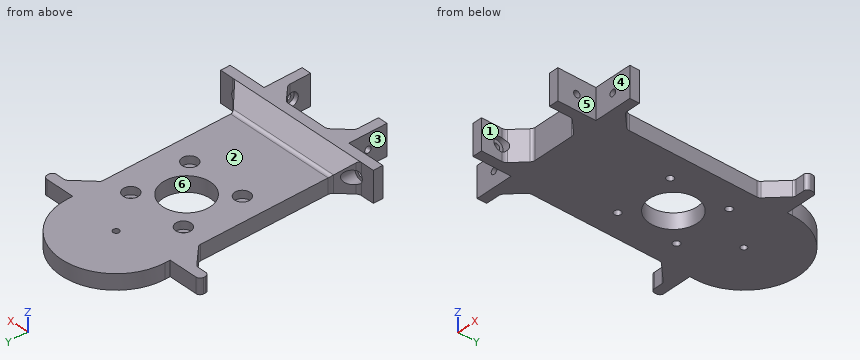
from build123d import *

# Parameters (mm, degrees)
RESSALTO_EXTRUS_O1_DEPTH                     = 8
RESSALTO_EXTRUS_O2_DEPTH                     = 8
CHANFRO1_SIZE                                = 8
ESBO_O3_R                                    = 1.6
ESBO_O3_R_2                                  = 12.5
CORTE_EXTRUS_O1_DEPTH                        = 138.275962936
FILETE1_R                                    = 3
REBAIXO_PARA_PARAFUSO_COM_CABE_A_PAN_2_COUNT = 2
REBAIXO_PARA_PARAFUSO_COM_CABE_A_PAN_2_PITCH = 70
CORTE_EXTRUS_O3_START                        = 10
ESBO_O13_R                                   = 3.5
CORTE_EXTRUS_O3_DEPTH                        = 10
ESBO_O18_R                                   = 3.5
CORTE_EXTRUS_O4_DEPTH                        = 2
ESBO_O19_R                                   = 1.8
CORTE_EXTRUS_O5_DEPTH                        = 137.574851278
ESBO_O20_R                                   = 4
CORTE_EXTRUS_O6_DEPTH                        = 4
ESBO_O21_W                                   = 17.35
ESBO_O21_H                                   = 5
RESSALTO_EXTRUS_O3_DEPTH                     = 8
FILETE2_R                                    = 2
CHANFRO2_SIZE                                = 10
FILETE3_R                                    = 2


with BuildPart() as part:
    # Esboço1 → Ressalto-extrusão1 (new body)
    with BuildSketch(Plane.XY):
        with BuildLine():
            Line((28.7, 5), (28.7, 100))
            ThreePointArc((28.7, 100), (0, 128.7), (-28.7, 100))
            Line((-28.7, 100), (-28.7, 5))
            Line((-28.7, 5), (-45, 5))
            Line((-45, 5), (-45, 0))
            Line((-45, 0), (-25, 0))
            Line((-25, 0), (-25, -20))
            Line((-25, -20), (-20, -20))
            Line((-20, -20), (-20, 0))
            Line((-20, 0), (20, 0))
            Line((20, 0), (20, -20))
            Line((20, -20), (25, -20))
            Line((25, -20), (25, 0))
            Line((25, 0), (45, 0))
            Line((45, 0), (45, 5))
            Line((45, 5), (28.7, 5))
        make_face()
    extrude(amount=RESSALTO_EXTRUS_O1_DEPTH)

    # Esboço2 → Ressalto-extrusão2 (add)
    with BuildSketch(Plane.XY.offset(8)):
        Polygon((-20, -20), (-25, -20), (-25, 0), (-45, 0), (-45, 5), (45, 5), (45, 0), (25, 0), (25, -20), (20, -20), (20, 0), (-20, 0), align=None)
    extrude(amount=RESSALTO_EXTRUS_O2_DEPTH)

    # Chanfro1
    chanfro1_edges = [part.edges().sort_by_distance(p)[0] for p in [
        (28.7, 5, 4),
        (20, 0, 8),
        (-20, 0, 8),
        (-28.7, 5, 4),
        (0, 5, 8),
    ]]
    chamfer(chanfro1_edges, length=CHANFRO1_SIZE - 0.0001)  # a hair under: the kernel refuses the full size

    # Esboço3 → Corte-extrusão1 (cut, through all)
    with BuildSketch(Plane(origin=(0, 0, 0), x_dir=(-1, 0, 0), z_dir=(0, 0, -1))):
        with Locations((0, 100)):
            Circle(ESBO_O3_R)
        with Locations((0, 63)):
            Circle(ESBO_O3_R_2)
    extrude(amount=-CORTE_EXTRUS_O1_DEPTH, mode=Mode.SUBTRACT)

    # Filete1
    filete1_edges = [part.edges().sort_by_distance(p)[0] for p in [
        (28.7, 12.9999, 4),
        (-36.6999, 5, 7.99995),
        (36.6999, 5, 7.99995),
        (-28.7, 12.9999, 4),
        (0, 12.9999, 8),
        (20, -7.9999, 8),
        (-12.0001, 0, 8),
        (12.0001, 0, 8),
        (-20, -7.9999, 8),
    ]]
    fillet(filete1_edges, radius=FILETE1_R)

    # Esboço12 → Rebaixo para parafuso com cabe_a panela (revolve, cut)
    with BuildSketch(Plane(origin=(35, 5, 8), x_dir=(0, 0, 1), z_dir=(1, 0, 0))):
        Polygon((0, 0), (0, 7.021463052), (1.7, 6), (1.7, 2.4), (3.5, 2.4), (3.5, 0), align=None)
    rebaixo_para_parafuso_com_cabe_a_panela = revolve(axis=Axis((35, 11.35, 8), (0, -1, 0)), mode=Mode.SUBTRACT)

    # Rebaixo para parafuso com cabe_a pan 2: Rebaixo para parafuso com cabe_a panela ×2
    with Locations(*[(-i * REBAIXO_PARA_PARAFUSO_COM_CABE_A_PAN_2_PITCH, 0, 0) for i in range(1, REBAIXO_PARA_PARAFUSO_COM_CABE_A_PAN_2_COUNT)]):
        add(rebaixo_para_parafuso_com_cabe_a_panela, mode=Mode.SUBTRACT)

    # Esboço13 → Corte-extrusão3 (cut)
    with BuildSketch(Plane(origin=(0, 5, 0), x_dir=(1, 0, 0), z_dir=(0, 1, 0)).offset(CORTE_EXTRUS_O3_START)):
        with Locations(Location((-35, -8, 0), (0, 0, 270))):
            Circle(ESBO_O13_R)
        with Locations(Location((35, -8, 0), (0, 0, 270))):
            Circle(ESBO_O13_R)
    extrude(amount=-CORTE_EXTRUS_O3_DEPTH, mode=Mode.SUBTRACT)

    # Esboço15 → Rebaixo para parafuso com cabe_a pan 3 (revolve, cut)
    with BuildSketch(Plane(origin=(20, -10, 8), x_dir=(0, 0, 1), z_dir=(0, 1, 0))):
        Polygon((0, 0), (0, 7.021463052), (1.7, 6), (1.7, 2.4), (3.5, 2.4), (3.5, 0), align=None)
    revolve(axis=Axis((13.65, -10, 8), (1, 0, 0)), mode=Mode.SUBTRACT)

    # Esboço17 → Rebaixo para parafuso com cabe_a pan 4 (revolve, cut)
    with BuildSketch(Plane(origin=(-20, -10, 8), x_dir=(0, 0, -1), z_dir=(0, 1, 0))):
        Polygon((0, 0), (0, 7.021463052), (1.7, 6), (1.7, 2.4), (3.5, 2.4), (3.5, 0), align=None)
    revolve(axis=Axis((-13.65, -10, 8), (-1, 0, 0)), mode=Mode.SUBTRACT)

    # Esboço18 → Corte-extrusão4 (cut)
    with BuildSketch(Plane.ZY.offset(-20)):
        with Locations((8, -10)):
            Circle(ESBO_O18_R)
    corte_extrus_o4 = extrude(amount=CORTE_EXTRUS_O4_DEPTH, mode=Mode.SUBTRACT)

    # Espelhar1: Corte-extrusão4 across plane
    add(corte_extrus_o4.mirror(Plane(origin=(0, 0, 0), x_dir=(0, 0, 1), z_dir=(1, 0, 0))), mode=Mode.SUBTRACT)

    # Esboço19 → Corte-extrusão5 (cut, through all)
    with BuildSketch(Plane.XY.offset(8)):
        with Locations((15.5, 78.5)):
            Circle(ESBO_O19_R)
        with Locations((15.5, 47.5)):
            Circle(ESBO_O19_R)
        with Locations((-15.5, 47.5)):
            Circle(ESBO_O19_R)
        with Locations((-15.5, 78.5)):
            Circle(ESBO_O19_R)
    extrude(amount=-CORTE_EXTRUS_O5_DEPTH, mode=Mode.SUBTRACT)

    # Esboço20 → Corte-extrusão6 (cut)
    with BuildSketch(Plane.XY.offset(8)):
        with Locations((15.5, 78.5)):
            Circle(ESBO_O20_R)
        with Locations((15.5, 47.5)):
            Circle(ESBO_O20_R)
        with Locations((-15.5, 47.5)):
            Circle(ESBO_O20_R)
        with Locations((-15.5, 78.5)):
            Circle(ESBO_O20_R)
    extrude(amount=-CORTE_EXTRUS_O6_DEPTH, mode=Mode.SUBTRACT)

    # Esboço21 → Ressalto-extrusão3 (add)
    with BuildSketch(Plane(origin=(0, 0, 0), x_dir=(-1, 0, 0), z_dir=(0, 0, -1))):
        with Locations((-37.375, 94.7)):
            Rectangle(ESBO_O21_W, ESBO_O21_H)
        with Locations((37.375, 94.7)):
            Rectangle(ESBO_O21_W, ESBO_O21_H)
    extrude(amount=-RESSALTO_EXTRUS_O3_DEPTH)

    # Filete2
    filete2_edges = [part.edges().sort_by_distance(p)[0] for p in [
        (46.05, 97.2, 4),
        (46.05, 92.2, 4),
        (-46.05, 92.2, 4),
        (-46.05, 97.2, 4),
    ]]
    fillet(filete2_edges, radius=FILETE2_R)

    # Chanfro2
    chanfro2_edges = [part.edges().sort_by_distance(p)[0] for p in [
        (28.7, 92.2, 4),
        (-28.7, 92.2, 4),
    ]]
    chamfer(chanfro2_edges, length=CHANFRO2_SIZE)

    # Filete3
    filete3_edges = [part.edges().sort_by_distance(p)[0] for p in [
        (38.7, 92.2, 4),
        (28.7, 82.2, 4),
        (-28.7, 82.2, 4),
        (-38.7, 92.2, 4),
    ]]
    fillet(filete3_edges, radius=FILETE3_R)


solid = part.part
Build history of the part. All positions in model axes, mm. Face numbers are marked on the shaded views. A direction names the side the tool comes from. Coordinates: 2 decimals unless noted, no trailing zeros. Write each loop counter-clockwise with the first axis right and the second up, starting at its lowest first coordinate (ties: lowest second). Pieces come first, ordered by that corner, then holes. Notation, with made-up numbers: (-7.75, 88.5) -> (47.25, 88.5) arc R25 ccw to (47.25, 108.5) -> close; hole circle Ø2 at (40.5, 39). An arc over 180 degrees is marked (long way). Use CSV: the item, a comma, the result in double quotes. Start each with the question number.
Q1. Cut at C-C, the plane y = 63. List the corners of the cut face in (x, z).
Q2. Pull direction Y, two halves, no side cores. Call the marked faces 4, 5 and 6: released by +Y, released by -Y, zero draft, split by the parting line, or undercut.
Q3. 3-axis set-ups, long thin cutter, end or side, ignore diameter. For the marked faces 1, 2 and 3: which of +Z, -Z, +X, -X, +Y, -Y reach the whole face in a straight line?
Q4. Cut at A-A, the plane y = 47.5. List the corners of the cut face in (x, z), then the cut area to 3 significant figures.
Q5. Flat gauge pins, fed straight in: pin 1 Ø5.5 at (y, z) = (2.5, 4) entering from +X; pin 2 Ø4 at (x, y) = (-29, 24) entering from +Z; pin 3 Ø5.5 at (x, z) = (-35, 8) entering from +Y. Where does each tip first touch, or does it go through?
Q6. Drill centre lines: probe 1 along X at (y, z) = (0.55, 8); probe 2 along X at (y, z) = (-12, 13.5); probe 3 along Z at (x, y) = (-35, 5). Where is each one in solid material? Low to high.
Q7. Cut at B-B, the plane x = 0. State how many separate pieces and enclosed holes the cut face has, then the cut area to 3 significant figures.
Checked values:
1,outline,"(-28.7, 0) -> (-12.5, 0) -> (-12.5, 8) -> (-28.7, 8) -> close; (12.5, 0) -> (28.7, 0) -> (28.7, 8) -> (12.5, 8) -> close"
2,face 4,"released by -Y"
2,face 5,"zero draft"
2,face 6,"undercut"
3,face 1,"+Z, -Z, -Y"
3,face 2,"+Z, +X, -X, +Y"
3,face 3,"+Z, -Z, -X, -Y"
4,outline,"(-28.7, 0) -> (-17.3, 0) -> (-17.3, 4) -> (-19.5, 4) -> (-19.5, 8) -> (-28.7, 8) -> close; (-13.7, 0) -> (13.7, 0) -> (13.7, 4) -> (11.5, 4) -> (11.5, 8) -> (-11.5, 8) -> (-11.5, 4) -> (-13.7, 4) -> close; (17.3, 0) -> (28.7, 0) -> (28.7, 8) -> (19.5, 8) -> (19.5, 4) -> (17.3, 4) -> close"
4,area,"366 mm²"
5,pin 1,"stops at x = 45"
5,pin 2,"stops at z = 8"
5,pin 3,"stops at y = 97.2"
6,probe 1,"x = -45 to -36.7, -33.3 to 33.3, 36.7 to 45"
6,probe 2,"x = -25 to -20, 20 to 25"
6,probe 3,"z = 0 to 4.5, 11.5 to 16"
7,separate pieces,"3"
7,enclosed holes,"0"
7,area,"876 mm²"
